from build123d import *

# Parameters (mm, degrees)
BOSS_EXTRUDE1_DEPTH = 3.175
BOSS_EXTRUDE2_DEPTH = 3.175
SKETCH3_W           = 6.236959702
SKETCH3_H           = 47.194711522
BOSS_EXTRUDE3_DEPTH = 3.175
SKETCH4_R           = 1.27
BOSS_EXTRUDE4_DEPTH = 3.175
BOSS_EXTRUDE5_REACH = 20.766
SKETCH6_W           = 1.202138058
SKETCH6_H           = 36.716281243
CUT_EXTRUDE1_REACH  = 11.525


with BuildPart() as part:
    # Sketch1 → Boss-Extrude1 (new body)
    with BuildSketch(Plane.XY):
        with BuildLine():
            Line((-17.114253333, -17.357583949), (-17.114253333, 17.357583949))
            ThreePointArc((-17.114253333, 17.357583949), (0, 24.432200125), (17.114253333, 17.357583949))
            Line((17.114253333, 17.357583949), (17.114253333, -17.357583949))
            ThreePointArc((17.114253333, -17.357583949), (0, -13.382802691), (-17.114253333, -17.357583949))
        make_face()
    extrude(amount=BOSS_EXTRUDE1_DEPTH)

    # Sketch2 → Boss-Extrude2 (add)
    with BuildSketch(Plane(origin=(0, 0, 0), x_dir=(-1, 0, 0), z_dir=(0, 0, -1))):
        with BuildLine():
            Line((-1.65128862, -13.417928303), (-1.65128862, 22.268343179))
            Line((-1.65128862, 22.268343179), (-1.65128862, 23.29835294))
            Line((-1.65128862, 23.29835294), (-2.853426735, 23.29835294))
            Line((-2.853426735, 23.29835294), (-2.853426735, -13.48778167))
            ThreePointArc((-2.853426735, -13.48778167), (-2.25262846, -13.448194961), (-1.65128862, -13.417928303))
        make_face()
        with BuildLine():
            Line((1.65128862, 23.29835294), (1.65128862, 22.268343179))
            Line((1.65128862, 22.268343179), (1.65128862, -13.417928303))
            ThreePointArc((1.65128862, -13.417928303), (2.25262846, -13.448194961), (2.853426735, -13.48778167))
            Line((2.853426735, -13.48778167), (2.853426735, 23.29835294))
            Line((2.853426735, 23.29835294), (1.65128862, 23.29835294))
        make_face()
    extrude(amount=BOSS_EXTRUDE2_DEPTH)

    # Sketch3 → Boss-Extrude3 (add)
    with BuildSketch(Plane.XY.offset(3.175)):
        with Locations((0, -23.258467244)):
            Rectangle(SKETCH3_W, SKETCH3_H)
    extrude(amount=-BOSS_EXTRUDE3_DEPTH)

    # Sketch4 → Boss-Extrude4 (add)
    with BuildSketch(Plane.XY.offset(3.175)):
        with Locations((0, -34.503683415)):
            Circle(SKETCH4_R)
    extrude(amount=BOSS_EXTRUDE4_DEPTH)

    # Sketch6 → Boss-Extrude5 (add, up to next)
    with BuildSketch(Plane.ZY.offset(-1.65128862), mode=Mode.PRIVATE) as boss_extrude5_sk1:
        with Locations((-2.573930971, 4.940212319)):
            Rectangle(SKETCH6_W, SKETCH6_H)
    boss_extrude5_tool1 = extrude(boss_extrude5_sk1.sketch, amount=BOSS_EXTRUDE5_REACH, mode=Mode.PRIVATE) - part.part
    add(boss_extrude5_tool1.solids().sort_by_distance((1.651289, 4.940212, -2.573931))[0])

    # Sketch8 → Cut-Extrude1 (cut, up to next)
    with BuildSketch(Plane(origin=(0, 0, -3.175), x_dir=(-1, 0, 0), z_dir=(0, 0, -1)), mode=Mode.PRIVATE) as cut_extrude1_sk1:
        Polygon((0, 23.29835294), (-0.889, 23.29835294), (-0.889, -13.417928303), (0.889, -13.417928303), (0.889, 23.29835294), align=None)
    cut_extrude1_tool1 = extrude(cut_extrude1_sk1.sketch, amount=-CUT_EXTRUDE1_REACH, mode=Mode.PRIVATE) & part.part
    add(cut_extrude1_tool1.solids().sort_by_distance((0, 4.940212, -3.175))[0], mode=Mode.SUBTRACT)


solid = part.part
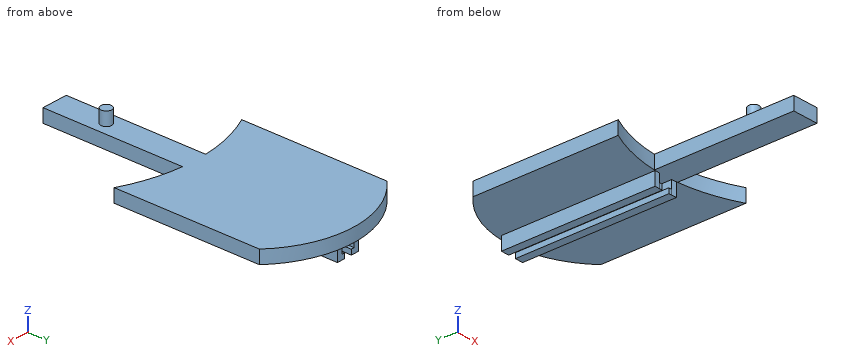
Model file for the job. Use its own axes, mm. Give positions to 0.01 mm unless a question says otherwise; leave off trailing zeros. Order: outer loops, then holes, each group sorted by start corner. A loop starts at its lowest first (then second) coordinate and runs counter-clockwise, first axis right, second up. Notation, with made-up numbers: (-20, -33) - (36, -33) arc R22 cw to (36, -7) - close; hole circle Ø4 at (10.5, 56). An arc over 180 degrees is marked (long way). Return JSON: item names as keys, results as strings.
1) Cut at C-C, the plane y = -15. Give the cut face in (x, z) (3 decimals), plus the area to 3 significant figures.
Geometry says:
{"outline": "(-17.114, 0) - (-11.09, 0) - (-11.09, 3.175) - (-17.114, 3.175) - close; (-3.118, 0) - (3.118, 0) - (3.118, 3.175) - (-3.118, 3.175) - close; (11.09, 0) - (17.114, 0) - (17.114, 3.175) - (11.09, 3.175) - close", "area": "58.1 mm²"}
2) Probe line 1 (X direction, y = -10.5, z = -2.25); line 2 (X direction, y = -6.5, z = -1.5); line 3 (Z direction, x = -2, y = 6) (3 decimals). List the from-to ranges inside material, lowest first. Write a range as from..to.
Geometry says:
{"line 1": "-2.85..-0.89, 0.89..2.85", "line 2": "-2.85..-1.65, 1.65..2.85", "line 3": "-3.175..3.175"}
3) Cut at D-D, the plane x = 0. Give the cut face in (y, z) (3 decimals), plus the area to 3 significant figures.
Geometry says:
{"outline": "(-46.856, 0) - (24.432, 0) - (24.432, 3.175) - (-33.234, 3.175) - (-33.234, 6.35) - (-35.774, 6.35) - (-35.774, 3.175) - (-46.856, 3.175) - close", "area": "234 mm²"}
4) Flat gauge pins, fed straight in: P1, Ø0.6, axis at x = 1, y = 2.5, coming from the +Z side (3 decimals); P2, Ø1, axis at x = 2.5, z = -1.5, coming from the +Y side; P3, Ø1.5, axis at x = -8.5, y = 13.5, coming from the -Z side. Where does each tip first touch, or does it go through?
Geometry says:
{"P1": "z = 3.175", "P2": "y = 23.3", "P3": "z = 0"}
5) Cut at A-A, the plane z = -0.75. Give the cut face in (x, y).
Geometry says:
{"outline": "(-2.85, -13.49) arc R38.83 cw to (-1.65, -13.42) - (-1.65, 23.3) - (-2.85, 23.3) - close; (1.65, -13.42) arc R38.83 cw to (2.85, -13.49) - (2.85, 23.3) - (1.65, 23.3) - close"}
6) Cut at B-B, the plane y = -4.5. Give the cut face in (x, z) (3 decimals).
Geometry says:
{"outline": "(-17.114, 0) - (-2.853, 0) - (-2.853, -3.175) - (-0.889, -3.175) - (-0.889, -1.973) - (-1.651, -1.973) - (-1.651, 0) - (1.651, 0) - (1.651, -1.973) - (0.889, -1.973) - (0.889, -3.175) - (2.853, -3.175) - (2.853, 0) - (17.114, 0) - (17.114, 3.175) - (-17.114, 3.175) - close"}
